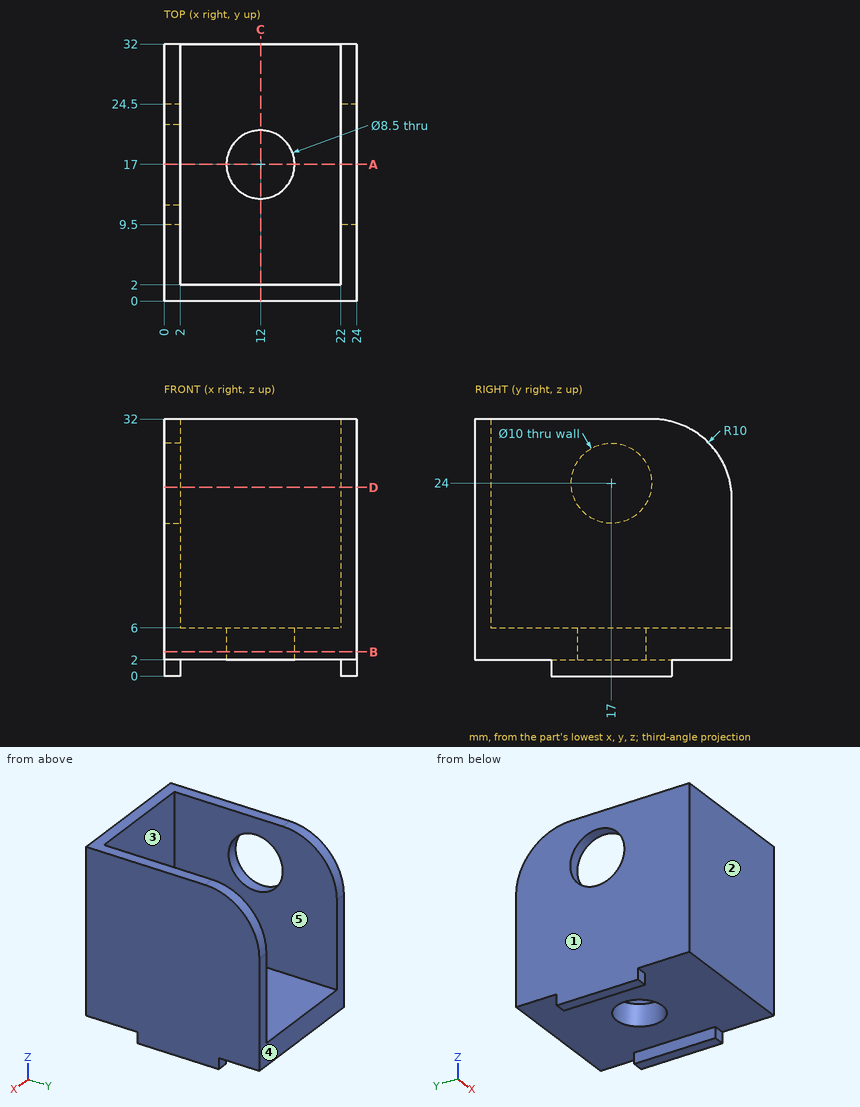
Input: dimensioned drawing with shaded views. Units: mm. Origin: part minimum x, y, z. A direction names the side the tool comes from. Coordinates: 2 decimals unless noted, no trailing zeros. Loops run counter-clockwise (first coordinate to the right, second up) from the corner with the lowest first, then second, coordinate; pieces in that order, holes last. Notation, with made-up numbers: M -12,67 L 39,67 A20 ccw 39,89 Z; hole C 87,26.25 d3. An arc over 180 degrees is marked long. Put each result on its own line as item: value.
(1) Access query for the marked faces 4 and 5. Directions: +Z, -Z, +X, -X, +Y, -Y. A direction counts if a zero-diameter tool reaches every point of the face in a straight line with its end or side. Return the directions, or none.
Answer sheet:
face 4: +Z, -Z, +X, -X, +Y
face 5: +Z, +Y
(2) Cut plane A-A on y = 17. Return the cut outline in (x, z), then the cut area to 3 significant figures.
Answer sheet:
outline: M 0,0 L 2,0 L 2,2 L 7.75,2 L 7.75,6 L 2,6 L 2,19 L 0,19 Z; M 0,29 L 2,29 L 2,32 L 0,32 Z; M 16.25,2 L 22,2 L 22,0 L 24,0 L 24,32 L 22,32 L 22,6 L 16.25,6 Z
area: 154 mm^2
(3) Cut plane C-C on x = 12. Return the cut outline in (y, z).
Answer sheet:
outline: M 0,2 L 12.75,2 L 12.75,6 L 2,6 L 2,32 L 0,32 Z; M 21.25,2 L 32,2 L 32,6 L 21.25,6 Z
(4) Cut plane B-B on z = 3. Return the cut outline in (x, y), then the cut area to 3 significant figures.
Answer sheet:
outline: M 0,0 L 24,0 L 24,32 L 0,32 Z; hole C 12,17 d8.5
area: 711 mm^2
(5) Cut plane D-D on z = 23.5. Return the cut outline in (x, y), then the cut area to 3 significant figures.
Answer sheet:
outline: M 0,0 L 24,0 L 24,31.89 L 22,31.89 L 22,2 L 2,2 L 2,12.03 L 0,12.03 Z; M 0,21.97 L 2,21.97 L 2,31.89 L 0,31.89 Z
area: 148 mm^2
(6) Material intervals for probe 1 along Y at (x, z) = (12, 3.85); probe 2 along X at (y, z) = (20.5, 30); probe 3 along Y at (x, z) = (20.75, 23), sorted ascending.
Answer sheet:
probe 1: y = 0 to 12.75, 21.25 to 32
probe 2: x = 0 to 2, 22 to 24
probe 3: y = 0 to 2
(7) First-contact query: pin 1 (1 mm diameter, centred on x = 23.5, z = 0.5, fed in from -Y); pin 2 (10 mm diameter, centred on x = 13, z = 23, fed in from +Y); pin 3 (10 mm diameter, centred on x = 11.5, y = 13, fed in from +Z); pin 4 (7 mm diameter, centred on x = 12, y = 17, fed in from +Z). Flat tips, straight axial feed; report the tip coordinate or a pass-through.
Answer sheet:
pin 1: stops at y = 9.5
pin 2: stops at y = 2
pin 3: stops at z = 6
pin 4: passes through
(8) Draft query along X for the marked faces 1, 2 and 3. Return one class per face: pulls with the +X half, pulls with the -X half, needs draft (parallel to the pull), parting line crosses it, or undercut.
Answer sheet:
face 1: pulls with the -X half
face 2: needs draft
face 3: undercut
